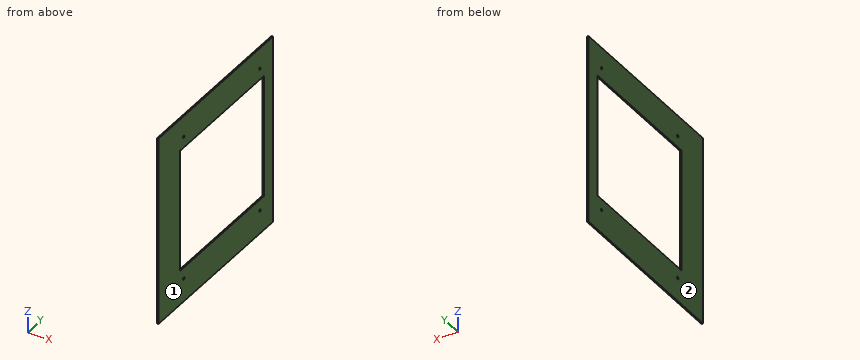
```python
from build123d import *

# Parameters (mm, degrees)
F0_W     = 374.65
F0_H     = 383.506636
F0_R     = 2.5
F0_W_2   = 274.65
F0_H_2   = 248.506636
F1_DEPTH = 3


with BuildPart() as f1:
    # F0 (on Right) → F1 (new body)
    with BuildSketch(Plane.YZ):
        with Locations((-20, -2.5)):
            Rectangle(F0_W, F0_H)
        with Locations((-124.61875, -146.84375)):
            Circle(F0_R, mode=Mode.SUBTRACT)
        with Locations((124.61875, -146.84375)):
            Circle(F0_R, mode=Mode.SUBTRACT)
        with Locations((-124.61875, 146.84375)):
            Circle(F0_R, mode=Mode.SUBTRACT)
        Rectangle(F0_W_2, F0_H_2, mode=Mode.SUBTRACT)
        with Locations((124.61875, 146.84375)):
            Circle(F0_R, mode=Mode.SUBTRACT)
    extrude(amount=F1_DEPTH)


solid = f1.part
```
Work out the finished part from the listing and answer in its coordinate system (mm). Face numbers are marked on the shaded views. Give positions to 0.01 mm unless a question says otherwise; leave off trailing zeros. Loops run counter-clockwise (first coordinate to the right, second up) from the corner with the lowest first, then second, coordinate; pieces in that order, holes last. Notation, with made-up numbers: (-32, 4) -> (12, 4) arc R19 ccw to (12, 32) -> close; hole circle Ø6 at (75, 56). An arc over 180 degrees is marked (long way). Use CSV: the item, a comma, the result in double quotes.
1. The part is cut by section A-A (z = 66.5). Write down the section's boundary in (x, y) (3 decimals), then the cut area to 3 significant figures.
Found:
outline,"(0, -207.325) -> (3, -207.325) -> (3, -137.325) -> (0, -137.325) -> close; (0, 137.325) -> (3, 137.325) -> (3, 167.325) -> (0, 167.325) -> close"
area,"300 mm^2"
2. Straight lines are drawn through the part: line 1 (Z direction, x = 2.35, y = 41); line 2 (Y direction, x = 2.3, z = -121) (3 decimals). For each, find the intervals that lie inside material, in ascending order.
Found:
line 1,"-194.25 to -124.25, 124.25 to 189.25"
line 2,"-207.325 to -137.325, 137.325 to 167.325"
3. The part is cut by section C-C (x = 0.55). Write down the section's boundary in (y, z) (3 decimals), then the cut area to 4 significant figures.
Found:
outline,"(-207.325, -194.253) -> (167.325, -194.253) -> (167.325, 189.253) -> (-207.325, 189.253) -> close; hole (-137.325, -124.253) -> (137.325, -124.253) -> (137.325, 124.253) -> (-137.325, 124.253) -> close; hole circle Ø5 at (-124.619, -146.844); hole circle Ø5 at (-124.619, 146.844); hole circle Ø5 at (124.619, -146.844); hole circle Ø5 at (124.619, 146.844)"
area,"75,350 mm^2"
4. The part is cut by section B-B (y = 86). Write down the section's boundary in (x, z), then the cut area to 3 significant figures.
Found:
outline,"(0, -194.25) -> (3, -194.25) -> (3, -124.25) -> (0, -124.25) -> close; (0, 124.25) -> (3, 124.25) -> (3, 189.25) -> (0, 189.25) -> close"
area,"405 mm^2"
5. The mould has two halves that part along X. Classify the marked faces 1 and 2: +X half, -X half, draft (parallel to the pull), parting line (faces both ways), or undercut.
Found:
face 1,"+X half"
face 2,"-X half"
